Autodesk Inventor part; units mm, degrees
ref_plane "YZ Plane" through (0, 0, 0) normal (1, 0, 0) x (0, 1, 0)
ref_plane "XZ Plane" through (0, 0, 0) normal (0, 1, 0) x (-1, 0, 0)
ref_plane "XY Plane" through (0, 0, 0) normal (0, 0, 1) x (1, 0, 0)
sketch "Sketch1" plane through (0, 0, 0) normal (0, 1, 0) x (-1, 0, 0)
  line L0 (9.8262, 5.9604) -> (-12.1738, 5.9604)
  line L1 (-12.1738, 5.9604) -> (-12.1738, -12.0396)
  line L2 (-12.1738, -12.0396) -> (9.8262, -12.0396)
  line L3 (9.8262, -12.0396) -> (9.8262, 5.9604)
  point P0 (0, 0)
  dimension "d0" = 22
  dimension "d1" = 18
extrude "Extrusion1" add sketch "Sketch1" along normal blind 3
sketch "Sketch2" plane through (-9.8262, 0, 5.9604) normal (0, 0, 1) x (1, 0, 0)
  line L0 (1, 2) -> (3, 2)
  line L1 (3, 2) -> (3, 1)
  line L2 (3, 1) -> (1, 1)
  line L3 (1, 1) -> (1, 2)
  line L4 (0, 3) -> (22, 3)
  line L5 (0, 0) -> (0, 3)
  line L6 (7, 2) -> (9, 2)
  line L7 (9, 2) -> (9, 1)
  line L8 (9, 1) -> (7, 1)
  line L9 (7, 1) -> (7, 2)
  line L10 (13, 2) -> (15, 2)
  line L11 (15, 2) -> (15, 1)
  line L12 (15, 1) -> (13, 1)
  line L13 (13, 1) -> (13, 2)
  line L14 (19, 2) -> (21, 2)
  line L15 (21, 2) -> (21, 1)
  line L16 (21, 1) -> (19, 1)
  line L17 (19, 1) -> (19, 2)
  line L18 (22, 0) -> (22, 3)
  point P0 (9.8262, 0)
  point P1 (1, 1.5)
  point P2 (7, 1.5)
  point P3 (13, 1.5)
  point P4 (19, 1.5)
  point P5 (8, 2)
  dimension "d4" = 1
  dimension "d5" = 1
  dimension "d6" = 2
  dimension "d7" = 1
  dimension "d8" = 1
  dimension "d9" = 2
  dimension "d10" = 1
  dimension "d11" = 2
  dimension "d12" = 1
  dimension "d13" = 2
  dimension "d14" = 1
  dimension "d15" = 1
  dimension "d16" = 1
  dimension "d17" = 1
  dimension "d18" = 4
  dimension "d19" = 4
extrude "Extrusion2" add sketch "Sketch2" along normal blind 18
sketch "Sketch3" plane through (0, 3, 0) normal (0, 1, 0) x (1, 0, 0)
  line L0 (12.1738, 12.0396) -> (9.1738, 12.0396)
  line L1 (12.1738, 12.0396) -> (-9.8262, 12.0396)
  line L2 (12.1738, 12.0396) -> (12.1738, 9.0396)
  line L3 (12.1738, 9.0396) -> (9.1738, 12.0396)
  point P0 (0, 0)
  dimension "d22" = 3
  dimension "d23" = 3
extrude "Extrusion3" cut sketch "Sketch3" against normal blind 18
properties part number "Rectifier"
Can you work these out from the model? Positions are in its coordinate system, mm. A direction names the side the tool comes from. Give positions to 0.01 mm unless a question says otherwise; leave off trailing zeros. Loops run counter-clockwise (first coordinate to the right, second up) from the corner with the lowest first, then second, coordinate; pieces in that order, holes last. Notation, with made-up numbers: (-34.75, -8.75) -> (21.25, -8.75) arc R15 cw to (21.25, 17.25) -> close; hole circle Ø7 at (55.25, 82). An arc over 180 degrees is marked (long way). Return JSON: item names as keys, results as strings.
Q1. I want a section at C-C, the plane y = 0.6. List the corners of the cut face in (x, z) for me, then the cut area to 4 significant figures.
Checks:
{"outline": "(-9.83, -12.04) -> (9.17, -12.04) -> (12.17, -9.04) -> (12.17, 5.96) -> (-9.83, 5.96) -> close", "area": "391.5 mm2"}
Q2. For pin 1 Ø1.1 at (y, z) = (1.5, 14.5) entering from +X; pin 2 Ø1.1 at (y, z) = (1.5, 11.5) entering from -X; pin 3 Ø0.6 at (x, z) = (3.5, 11) entering from -Y, each with a flat end and sliding along its axis, tell me the tip position at first contact or that it passes through.
Checks:
{"pin 1": "stops at x = 11.17", "pin 2": "stops at x = -8.83", "pin 3": "stops at y = 1"}
Q3. I need wall thicknesses on probe 1 along X at (y, z) = (1.4, 19); probe 2 along Z at (x, y) = (8, 1.25); probe 3 along Y at (x, z) = (-1.5, 22). Which ranges of each line are inside material? Lowest first, please.
Checks:
{"probe 1": "x = -8.83 to -6.83, -2.83 to -0.83, 3.17 to 5.17, 9.17 to 11.17", "probe 2": "z = -12.04 to 5.96", "probe 3": "y = 1 to 2"}
Q4. On a 3-axis mill with a long thin cutter (end or side, diameter ignored), from which of +Z, -Z, +X, -X, +Y, -Y can I reach the whole of each face in a straight line? I mean faces 5 (the face through (-8.826, 1.5, 14.8)), 6 (the face through (4, 1, 15)), 7 (the face through (4, 2, 15)), 8 (the face through (1, 3, -3)), 9 (the face through (9.174, 1.5, 14.8)). Say none if no direction works.
Checks:
{"face 5": "+Z, -X, +Y, -Y", "face 6": "+Z, +X, -X, -Y", "face 7": "+Z, +X, -X, +Y", "face 8": "+Z, -Z, +X, -X, +Y", "face 9": "+Z, +Y, -Y"}
Q5. I want a section at A-A, the plane z = 11.5. List the corners of the cut face in (x, y) for me.
Checks:
{"outline": "(-8.83, 1) -> (-6.83, 1) -> (-6.83, 2) -> (-8.83, 2) -> close; (-2.83, 1) -> (-0.83, 1) -> (-0.83, 2) -> (-2.83, 2) -> close; (3.17, 1) -> (5.17, 1) -> (5.17, 2) -> (3.17, 2) -> close; (9.17, 1) -> (11.17, 1) -> (11.17, 2) -> (9.17, 2) -> close"}
Q6. I want a section at D-D, the plane x = 8.25. List the corners of the cut face in (y, z) for me, then the cut area to 3 significant figures.
Checks:
{"outline": "(0, -12.04) -> (3, -12.04) -> (3, 5.96) -> (0, 5.96) -> close", "area": "54.0 mm2"}
Q7. We'd pull the mould along X, two halves only. Please class faces 1 (the face through (-0.826, 1.5, 14.8)), 2 (the face through (-9.826, 1, -3)), 3 (the face through (-6.826, 1.5, 14.8)), 4 (the face through (10, 1, 15)): released by +X, released by -X, zero draft, split by the parting line, or undercut.
Checks:
{"face 1": "undercut", "face 2": "released by -X", "face 3": "undercut", "face 4": "zero draft"}
Q8. I want a section at B-B, the plane x = -7.25. List the corners of the cut face in (y, z) for me.
Checks:
{"outline": "(0, -12.04) -> (3, -12.04) -> (3, 5.96) -> (2, 5.96) -> (2, 23.96) -> (1, 23.96) -> (1, 5.96) -> (0, 5.96) -> close"}
